Could you check a few things on this model? Use its own coordinates, in mm. A direction names the side the tool comes from. Coordinates: 2 decimals unless noted, no trailing zeros. Order: outer loops, then holes, each group sorted by start corner. A loop starts at its lowest first (then second) coordinate and runs counter-clockwise, first axis right, second up. Notation, with made-up numbers: (16.5, 77.25) -> (28.5, 77.25) arc R30 ccw to (28.5, 99.25) -> close; hole circle Ø7 at (85, 59.5). An arc over 180 degrees is marked (long way). Put each result on its own line as item: value. Start each with the question number.
Q1. Please list where these lines run through material, in increasing order: line 1 along Z through (x, y) = (11.4, 73.5); line 2 along Y through (x, z) = (12.4, -49.5); line 3 along Y through (x, z) = (15, -43.5).
Q2. For faces 4 (the face through (13, 104.26, -48)), 5 (the face through (11, 42, -63)), which set-ups out of +Z, -Z, +X, -X, +Y, -Y let a thin tool reach every point of the face, with its end or its side?
Q3. If we section it at A-A (x = 15.25): Count the separate pieces of the cut face and the enclosed holes in it, and give its area (3 significant figures).
Q4. If we section it at C-C (z = -35): Please give me the cut outline in (x, y).
Q5. Will these pins go through, and if not, where does the flat tip stop? pin 1 (1 mm diameter, centred on y = 74.5, z = -68.5, fed in from +X); pin 2 (5.5 mm diameter, centred on y = 52.51, z = -44.25, fed in from +X); pin 3 (3 mm diameter, centred on x = 13, y = 47, fed in from +Z).
Q6. If we section it at D-D (y = 85): Please give me the cut outline in (x, z).
Q7. We'd pull the mould along Z, two halves only. Please class faces 1 (the face through (13.535, 103.828, -23.153)), 2 (the face through (13, 40.01, -55)), 3 (the face through (13, 61, -34.074)): +Z half, -Z half, draft (parallel to the pull), parting line (faces both ways), or undercut.
Q8. If we section it at B-B (y = 52.51): Please give me the cut outline in (x, z), and give its area (3 significant figures).
from build123d import *

# Parameters (mm, degrees)
PAD011_DEPTH         = 6
POCKET011_DEPTH      = 4.5
POCKET011_DEPTH_BACK = 100
SKETCH030_R          = 1.6
POCKET013_DEPTH      = 5


with BuildPart() as part:
    # CopySketch028 → Pad011 (new body)
    with BuildSketch(Plane.YZ):
        with BuildLine():
            Line((69.62, -34.0739220052), (104.26, -20.95))
            Line((104.26, -20.95), (104.26, -75.95))
            Line((104.26, -75.95), (40.01, -64.8058991482))
            Line((40.01, -64.8058991482), (40.01, -44.4358991482))
            ThreePointArc((53.3737933734, -34.0739220052), (44.4834146169, -36.4066415985), (40.01, -44.4358991482))
            Line((53.3737933734, -34.0739220052), (69.62, -34.0739220052))
        make_face()
    extrude(amount=PAD011_DEPTH)

    # Sketch028 → Pocket011 (cut, two sides)
    with BuildSketch(Plane.YZ.offset(6)) as pocket011_sk:
        with BuildLine():
            ThreePointArc((54.3211015793, -41.1506327381), (48.924493396, -44.0759059246), (54.0123107229, -47.5102498135))
            Line((54.0123107229, -47.5102498135), (70.19, -46.8041455781))
            Line((70.19, -46.8041455781), (70.19, -42.8041455781))
            Line((70.19, -42.8041455781), (54.3211015793, -41.1506327381))
        make_face()
    extrude(amount=-POCKET011_DEPTH, mode=Mode.SUBTRACT)
    extrude(pocket011_sk.sketch, amount=POCKET011_DEPTH_BACK, mode=Mode.SUBTRACT)

    # Sketch030 (on Face5 of Pocket011) → Pocket013 (cut)
    with BuildSketch(Plane.YZ.offset(6)):
        with Locations((74.898643, -48.273617)):
            Circle(SKETCH030_R)
        with Locations((74.845955, -34.282856)):
            Circle(SKETCH030_R)
        with Locations((102.302101, -23.633244)):
            Circle(SKETCH030_R)
        with Locations((102.323669, -48.271477)):
            Circle(SKETCH030_R)
        with Locations((102.305855, -72.383957)):
            Circle(SKETCH030_R)
        with Locations((74.864891, -68.281929)):
            Circle(SKETCH030_R)
        with Locations((41.8248800985, -63.330712397)):
            Circle(SKETCH030_R)
    extrude(amount=-POCKET013_DEPTH, mode=Mode.SUBTRACT)


with BuildPart() as part_1:
    # Body004 placement: moved
    add(part.part.moved(Location((10, 0, 0))))


solid = part_1.part
The answers:
1. line 1: -70.61 to -69.12, -67.45 to -49.05, -47.5 to -35.15, -33.42 to -32.6
1. line 2: 40.01 to 73.87, 75.93 to 101.3, 103.35 to 104.26
1. line 3: 40.15 to 49, 70.19 to 104.26
2. face 4: +Z, -Z, +X, -X, +Y
2. face 5: +X
3. separate pieces: 1
3. enclosed holes: 8
3. area: 2,360 mm^2
4. outline: (10, 46.81) -> (16, 46.81) -> (16, 73.42) -> (11, 73.42) -> (11, 76.28) -> (16, 76.28) -> (16, 104.26) -> (10, 104.26) -> close
5. pin 1: x = 11
5. pin 2: x = 11.5
5. pin 3: z = -34.38
6. outline: (10, -72.61) -> (16, -72.61) -> (16, -28.25) -> (10, -28.25) -> close
7. face 1: undercut
7. face 2: draft
7. face 3: +Z half
8. outline: (10, -66.97) -> (16, -66.97) -> (16, -47.84) -> (11.5, -47.84) -> (11.5, -40.66) -> (16, -40.66) -> (16, -33.98) -> (10, -33.98) -> close
8. area: 166 mm^2
